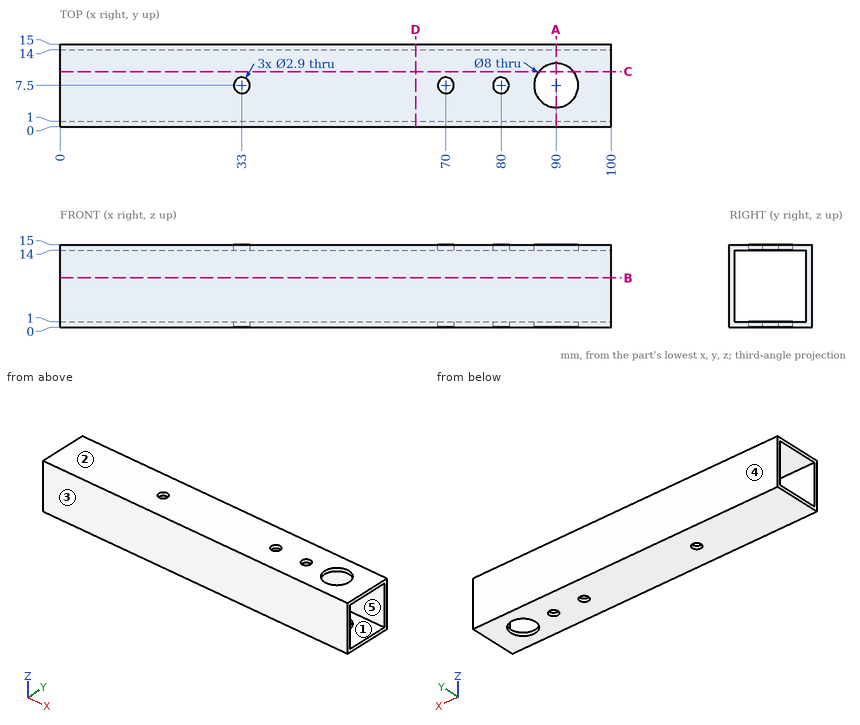
Can you work these out from the drawing? Everything is in mm from the part's minimum corner. A direction names the side the tool comes from. Round coordinates to 2 decimals unless told otherwise and drop trailing zeros. Order: outer loops, then holes, each group sorted by start corner. A loop starts at its lowest first (then second) coordinate and runs counter-clockwise, first axis right, second up. Notation, with made-up numbers: (4, 66) - (13, 66) arc R9 cw to (13, 70) - close; hole circle Ø9 at (-5.75, 84). An arc over 180 degrees is marked (long way). Answer in a Markdown table with one row per item.
(1) Suppose I cut it at B-B, the plane z = 9. Please give me the cut outline in (x, y), plus the area to 3 significant figures.
From the geometry:
| item | result |
|---|---|
| outline | (0, 0) - (100, 0) - (100, 1) - (0, 1) - close; (0, 14) - (100, 14) - (100, 15) - (0, 15) - close |
| area | 200 mm2 |
(2) Suppose I cut it at C-C, the plane y = 10. Please give me the cut outline in (x, z).
From the geometry:
| item | result |
|---|---|
| outline | (0, 0) - (86.88, 0) - (86.88, 1) - (0, 1) - close; (0, 14) - (86.88, 14) - (86.88, 15) - (0, 15) - close; (93.12, 0) - (100, 0) - (100, 1) - (93.12, 1) - close; (93.12, 14) - (100, 14) - (100, 15) - (93.12, 15) - close |
(3) For P1, Ø1.7, axis at x = 70, y = 7.5, coming from the +Z side, with a flat end and sliding along its axis, tell me the tip position at first contact or that it passes through.
From the geometry:
| item | result |
|---|---|
| P1 | passes through |
(4) Suppose I cut it at A-A, the plane x = 90. Please give me the cut outline in (y, z).
From the geometry:
| item | result |
|---|---|
| outline | (0, 0) - (3.5, 0) - (3.5, 1) - (1, 1) - (1, 14) - (3.5, 14) - (3.5, 15) - (0, 15) - close; (11.5, 0) - (15, 0) - (15, 15) - (11.5, 15) - (11.5, 14) - (14, 14) - (14, 1) - (11.5, 1) - close |
(5) Which directions (+Z, -Z, +X, -X, +Y, -Y) give clear straight access to the entire face, cutting with the end or side of a thin tool? Please do the marked faces 4 and 5.
From the geometry:
| item | result |
|---|---|
| face 4 | +Z, -Z, +X, -X, +Y |
| face 5 | +X, -X |
(6) Suppose I cut it at D-D, the plane x = 64.5. Please give me the cut outline in (y, z), plus the area to 3 significant figures.
From the geometry:
| item | result |
|---|---|
| outline | (0, 0) - (15, 0) - (15, 15) - (0, 15) - close; hole (1, 1) - (14, 1) - (14, 14) - (1, 14) - close |
| area | 56.0 mm2 |
(7) If we mould it in two halves opening along Z, with no side actions, what happens to the marked faces 1, 2 and 3? For each: released by +Z, released by -Z, zero draft, split by the parting line, or undercut.
From the geometry:
| item | result |
|---|---|
| face 1 | undercut |
| face 2 | released by +Z |
| face 3 | zero draft |
(8) Please list where these lines run through material, in increasing order: L1, parallel to Y at x = 41, z = 5.5; L2, parallel to Y at x = 80, z = 14.7. Write a range as from..to.
From the geometry:
| item | result |
|---|---|
| L1 | y = 0..1, 14..15 |
| L2 | y = 0..6.05, 8.95..15 |
